Read the model definition and answer for the solid it produces. Units are mm, in the model's axes. A direction names the side the tool comes from. Give positions to 0.01 mm unless a question says otherwise; leave off trailing zeros. Order: outer loops, then holes, each group sorted by start corner. A loop starts at its lowest first (then second) coordinate and runs counter-clockwise, first axis right, second up.
Item 1: Which of the six approach directions +Z, -Z, +X, -X, +Y, -Y give full straight-line access (tool end or side, diameter ignored) to faces 5 (the face through (10.565, 13, 3)), 6 (the face through (89.615, -2, 3)), 7 (the face through (-29.3, 30.67, 2.96)), 8 (the face through (102, 0, 3)), 9 (the face through (0, 3, 3))?
Item 2: A cutting plane is placed at C-C (x = -18). Write down the section's boundary in (y, z), plus the area to 3 significant figures.
Item 3: Find the intervals of material crossed by line 1 along X through (y, z) = (-2, 2.25); line 2 along X through (y, z) = (15.5, 1.7); line 3 along Y through (x, z) = (27.5, 0.8), in increasing order.
Item 4: A cutting plane is placed at B-B (y = 18.5). Write down the section's boundary in (x, z), plus the area to 3 significant figures.
Item 5: Given pin 1 Ø1.8 at (x, z) = (73.5, 3.5) entering from +Y; pin 2 Ø1 at (y, z) = (11.5, 1) entering from +X; pin 3 Ø1.2 at (y, z) = (-1.5, 3) entering from +X, each flat-ended and moving along its own axis, determine where each tip first touches the part or whether it passes through.
Item 6: The mould has two halves that part along Y. Classify faces 1 (the face through (78.565, 13, 3)), 2 (the face through (13.615, -2, 3)), 3 (the face through (118.3, 30.8, 3)), 4 (the face through (40.565, 13, 3)): +Y half, -Y half, draft (parallel to the pull), parting line (faces both ways), or undercut.
Item 7: A cutting plane is placed at A-A (x = 72.5). Write down the section's boundary in (y, z).
Item 8: A cutting plane is placed at D-D (z = 2.1). State how many separate pieces and enclosed holes the cut face has, plus the area to 3 significant figures.
Autodesk Inventor part; units mm, degrees
ref_plane "YZ Plane" through (0, 0, 0) normal (1, 0, 0) x (0, 1, 0)
ref_plane "XZ Plane" through (0, 0, 0) normal (0, 1, 0) x (-1, 0, 0)
ref_plane "XY Plane" through (0, 0, 0) normal (0, 0, 1) x (1, 0, 0)
sketch "Sketch1" plane through (0, 0, 0) normal (0, 0, 1) x (1, 0, 0)
  circle A0 centre (-18.4853, 20.4853) radius 4.25
  circle A1 centre (107.6147, 20.4853) radius 4.25
  line L0 (-33.4853, 26.4853) -> (-33.4853, 14.4853)
  line L1 (-33.4853, 26.4853) -> (-25, 34.9706)
  line L2 (-33.4853, 14.4853) -> (-25, 6)
  line L3 (-25, 34.9706) -> (114.1294, 34.9706)
  line L4 (114.1294, 34.9706) -> (122.6147, 26.4853)
  line L5 (122.6147, 26.4853) -> (122.6147, 14.4853)
  line L6 (122.6147, 14.4853) -> (114.1294, 6)
  circle A2 centre (-18.4853, 20.4853) radius 13 construction
  circle A3 centre (-18.4853, 20.4853) radius 17 construction
  line L7 (-25, 6) -> (0, 6)
  line L8 (0, 6) -> (0, 0)
  line L9 (114.1294, 6) -> (105.6147, 6)
  line L10 (105.6147, 6) -> (105.6147, 0)
  line L11 (105.6147, 0) -> (0, 0)
  point P0 (0, 0)
  point P1 (-33.4853, 20.4853)
  dimension "d0" = 8.5
  dimension "d1" = 126.1
  dimension "d2" = 45
  dimension "d3" = 12
  dimension "d4" = 26
  dimension "d5" = 34
  dimension "d6" = 15
  dimension "d7" = 6
  dimension "d10" = 15
  dimension "d18" = 2
  dimension "d19" = 25
extrude "Extrusion1" add sketch "Sketch1" along normal blind 6
sketch "Sketch2" plane through (0, 0, 6) normal (0, 0, 1) x (1, 0, 0)
  line L0 (114.1294, 34.9706) -> (-25, 34.9706)
  line L1 (-25, 34.9706) -> (-33.4853, 26.4853)
  line L2 (-13, 34.9706) -> (-4.5147, 26.4853)
  line L3 (-4.5147, 26.4853) -> (93.6442, 26.4853)
  line L4 (93.6442, 26.4853) -> (102.1294, 34.9706)
  point P0 (-33.4853, 14.4853)
  dimension "d13" = 12
  dimension "d14" = 12
  dimension "d15" = 12
extrude "Extrusion2" cut sketch "Sketch2" against normal blind 6
sketch "Sketch3" plane through (0, 0, 6) normal (0, 0, 1) x (1, 0, 0)
  line L0 (0, 0) -> (105.6147, 0)
  line L1 (93.6442, 26.4853) -> (-4.5147, 26.4853)
  line L2 (40.5647, 16) -> (48.5647, 16)
  line L3 (48.5647, 16) -> (48.5647, 10)
  line L4 (48.5647, 10) -> (40.5647, 10)
  line L5 (40.5647, 10) -> (40.5647, 16)
  line L6 (10.5647, 16) -> (18.5647, 16)
  line L7 (18.5647, 16) -> (18.5647, 10)
  line L8 (18.5647, 10) -> (10.5647, 10)
  line L9 (10.5647, 10) -> (10.5647, 16)
  line L10 (70.5647, 16) -> (78.5647, 16)
  line L11 (78.5647, 16) -> (78.5647, 10)
  line L12 (78.5647, 10) -> (70.5647, 10)
  line L13 (70.5647, 10) -> (70.5647, 16)
  point P0 (44.5647, 16)
  point P1 (44.5647, 26.4853)
  dimension "d20" = 8
  dimension "d21" = 6
  dimension "d22" = 8
  dimension "d23" = 8
  dimension "d24" = 10
  dimension "d25" = 22
  dimension "d26" = 22
extrude "Extrusion3" cut sketch "Sketch3" against normal through all
sketch "Sketch4" plane through (0, 0, 6) normal (0, 0, 1) x (1, 0, 0)
  line L0 (0, 0) -> (105.6147, 0)
  line L1 (97.6147, 0) -> (89.6147, 0)
  line L2 (89.6147, 0) -> (89.6147, -4)
  line L3 (91.6147, -6) -> (95.6147, -6)
  line L4 (97.6147, -4) -> (97.6147, 0)
  line L5 (64.6147, 0) -> (56.6147, 0)
  line L6 (56.6147, 0) -> (56.6147, -4)
  line L7 (58.6147, -6) -> (62.6147, -6)
  line L8 (64.6147, -4) -> (64.6147, 0)
  line L9 (21.6147, 0) -> (13.6147, 0)
  line L10 (13.6147, 0) -> (13.6147, -4)
  line L11 (15.6147, -6) -> (19.6147, -6)
  line L12 (21.6147, -4) -> (21.6147, 0)
  arc A0 (13.6147, -4) -> (15.6147, -6) centre (15.6147, -4) ccw
  arc A1 (19.6147, -6) -> (21.6147, -4) centre (19.6147, -4) ccw
  arc A2 (56.6147, -4) -> (58.6147, -6) centre (58.6147, -4) ccw
  arc A3 (62.6147, -6) -> (64.6147, -4) centre (62.6147, -4) ccw
  arc A4 (89.6147, -4) -> (91.6147, -6) centre (91.6147, -4) ccw
  arc A5 (95.6147, -6) -> (97.6147, -4) centre (95.6147, -4) ccw
  dimension "d29" = 2
  dimension "d30" = 8
  dimension "d31" = 8
  dimension "d32" = 8
  dimension "d33" = 6
  dimension "d34" = 8
  dimension "d35" = 25
  dimension "d36" = 35
extrude "Extrusion4" add sketch "Sketch4" against normal blind 6
chamfer "Chamfer1" distance 2 angle 45 1 edges at (105.6147, 6, 3)
equation "\"d14\" = d13"
equation "\"d15\" = d14"
equation "\"d26\" = d25"
properties part number "rope_mount_a"
Response values:
1. face 5: +Z, -Z
1. face 6: +Z, -Z, -Y
1. face 7: +Z, -Z, -X, +Y
1. face 8: +Z, -Z, +X, -Y
1. face 9: +Z, -Z, -X, -Y
2. outline: (6, 0) - (16.26, 0) - (16.26, 6) - (6, 6) - close; (24.71, 0) - (34.97, 0) - (34.97, 6) - (24.71, 6) - close
2. area: 123 mm2
3. line 1: x = 13.61 to 21.61, 56.61 to 64.61, 89.61 to 97.61
3. line 2: x = -33.49 to 10.56, 18.56 to 40.56, 48.56 to 70.56, 78.56 to 122.61
3. line 3: y = 0 to 26.49
4. outline: (-33.49, 0) - (-22.24, 0) - (-22.24, 6) - (-33.49, 6) - close; (-14.73, 0) - (103.86, 0) - (103.86, 6) - (-14.73, 6) - close; (111.37, 0) - (122.61, 0) - (122.61, 6) - (111.37, 6) - close
4. area: 846 mm2
5. pin 1: stops at y = 26.49
5. pin 2: stops at x = 120.13
5. pin 3: stops at x = 97.61
6. face 1: undercut
6. face 2: draft
6. face 3: +Y half
6. face 4: undercut
7. outline: (0, 0) - (10, 0) - (10, 6) - (0, 6) - close; (16, 0) - (26.49, 0) - (26.49, 6) - (16, 6) - close
8. separate pieces: 1
8. enclosed holes: 5
8. area: 3,990 mm2
